The drawing under review shows one solid part. Ordinate dimensions are in mm from its lowest x, y, z. Give positions to 0.01 mm unless a question says otherwise; leave off trailing zeros. Write each loop counter-clockwise with the first axis right and the second up, starting at its lowest first coordinate (ties: lowest second). Pieces come first, ordered by that corner, then holes.
Q1. We need section C-C (x = 2). Write out the cut boundary in (y, z), then the cut area to 3 significant figures.
Q2. Insertion check: P1, Ø1.8, axis at x = 21.862, z = 23, coming from the +Y side. The pin has a flat end and moves straight along its axis. Give the tip position at first contact, or say it passes through.
Q3. We need section A-A (z = 10.5). Write out the cut boundary in (x, y).
Q4. For line 1 (X direction, y = 0.7, z = 10.5); line 2 (X direction, y = 0.75, z = 23); line 3 (Z direction, x = 2, y = 0.85), list the stretches that pass through material, from the lowest coordinate up.
Q5. We need section B-B (y = 0.9). Write out the cut boundary in (x, z), then the cut area to 3 significant figures.
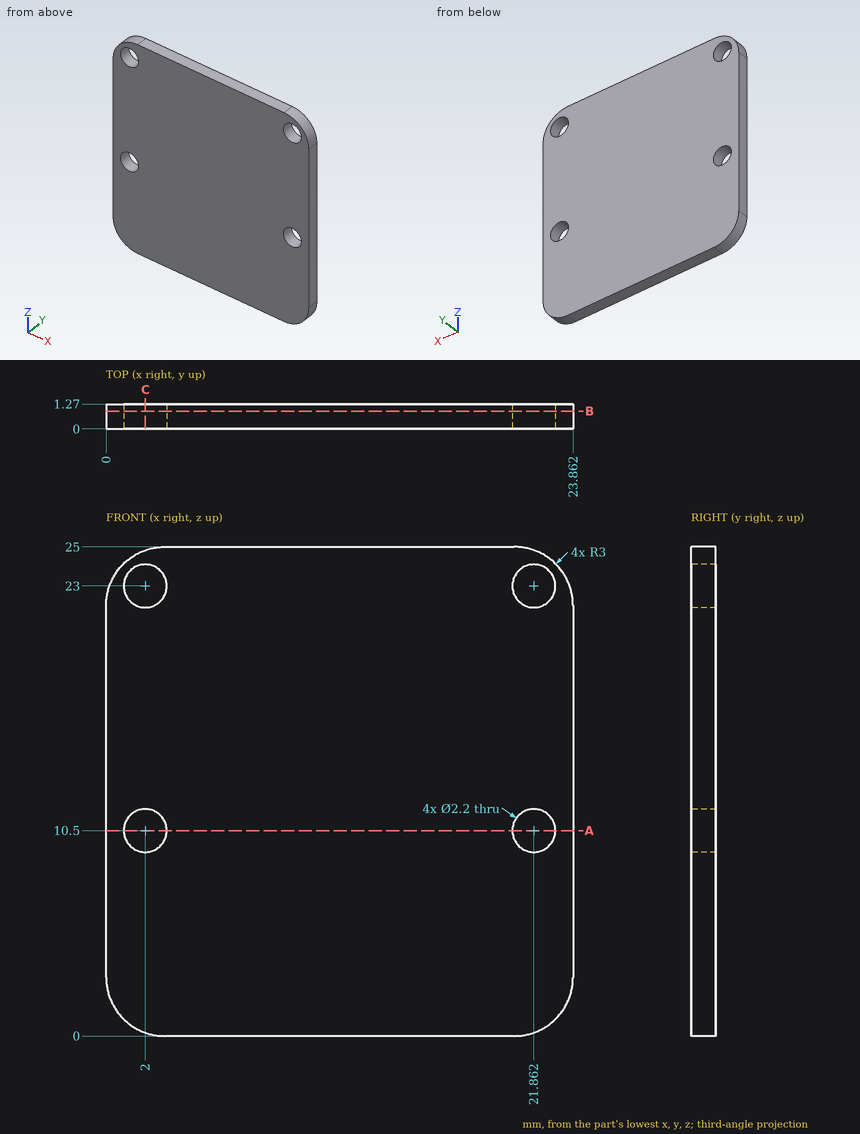
Computed:
1. outline: (0, 0.17) - (1.27, 0.17) - (1.27, 9.4) - (0, 9.4) - close; (0, 11.6) - (1.27, 11.6) - (1.27, 21.9) - (0, 21.9) - close; (0, 24.1) - (1.27, 24.1) - (1.27, 24.83) - (0, 24.83) - close
1. area: 25.7 mm2
2. P1: passes through
3. outline: (0, 0) - (0.9, 0) - (0.9, 1.27) - (0, 1.27) - close; (3.1, 0) - (20.76, 0) - (20.76, 1.27) - (3.1, 1.27) - close; (22.96, 0) - (23.86, 0) - (23.86, 1.27) - (22.96, 1.27) - close
4. line 1: x = 0 to 0.9, 3.1 to 20.76, 22.96 to 23.86
4. line 2: x = 0.17 to 0.9, 3.1 to 20.76, 22.96 to 23.69
4. line 3: z = 0.17 to 9.4, 11.6 to 21.9, 24.1 to 24.83
5. outline: (0, 3) arc R3 ccw to (3, 0) - (20.86, 0) arc R3 ccw to (23.86, 3) - (23.86, 22) arc R3 ccw to (20.86, 25) - (3, 25) arc R3 ccw to (0, 22) - close; hole circle Ø2.2 at (2, 10.5); hole circle Ø2.2 at (2, 23); hole circle Ø2.2 at (21.86, 10.5); hole circle Ø2.2 at (21.86, 23)
5. area: 574 mm2
